from build123d import *

# Parameters (mm, degrees)
SKETCH1_R            = 2.5
SKETCH1_W            = 0.25
SKETCH1_H            = 1
SKETCH1_R_2          = 0.5
BOSS_EXTRUDE1_DEPTH  = 15
SKETCH1_3_R          = 2.5
SKETCH1_3_R_2        = 0.5
BOSS_EXTRUDE2_DEPTH  = 0.8
SKETCH1_5_W          = 0.25
SKETCH1_5_H          = 1
BOSS_EXTRUDE3_DEPTH  = 1.5
SKETCH2_R            = 0.200548898
CUT_EXTRUDE3_DEPTH   = 1.5
BOSS_EXTRUDE4_DEPTH  = 0.5
BOSS_EXTRUDE6_START  = 3
BOSS_EXTRUDE6_DEPTH  = 0.5
SKETCH6_R            = 1.35
BOSS_EXTRUDE7_DEPTH  = 8
BOSS_EXTRUDE9_START  = 4.5
SKETCH9_R            = 0.5
SKETCH9_R_2          = 1.5
BOSS_EXTRUDE9_DEPTH  = 0.5
SKETCH10_R           = 2
SKETCH10_R_2         = 1.5
BOSS_EXTRUDE10_DEPTH = 0.5
FILLET1_R            = 0.5
BOSS_EXTRUDE11_START = -0.5
SKETCH11_R           = 1.5
BOSS_EXTRUDE11_DEPTH = 0.5


with BuildPart() as part:
    # Sketch1 → Boss-Extrude1 (new body)
    # profile 1 of 5: a face of its own
    with BuildSketch(Plane(origin=(0, 0, 0), x_dir=(1, 0, 0), z_dir=(0, 1, 0))):
        with BuildLine():
            Line((-3.31662479, -5), (3.31662479, -5))
            ThreePointArc((3.31662479, -5), (6, 0), (3.31662479, 5))
            Line((3.31662479, 5), (-3.31662479, 5))
            ThreePointArc((-3.31662479, 5), (-6, 0), (-3.31662479, -5))
        make_face()
        Circle(SKETCH1_R, mode=Mode.SUBTRACT)
        with Locations((4, 0)):
            Rectangle(SKETCH1_W, SKETCH1_H, mode=Mode.SUBTRACT)
        with Locations((-4, 0)):
            Rectangle(SKETCH1_W, SKETCH1_H, mode=Mode.SUBTRACT)
    # profile 2 of 5: a face of its own
    with BuildSketch(Plane(origin=(0, 0, 0), x_dir=(1, 0, 0), z_dir=(0, 1, 0))):
        Circle(SKETCH1_R)
        Circle(SKETCH1_R_2, mode=Mode.SUBTRACT)
    # profile 3 of 5: a face of its own
    with BuildSketch(Plane(origin=(0, 0, 0), x_dir=(1, 0, 0), z_dir=(0, 1, 0))):
        with Locations((-4, 0)):
            Rectangle(SKETCH1_W, SKETCH1_H)
    # profile 4 of 5: a face of its own
    with BuildSketch(Plane(origin=(0, 0, 0), x_dir=(1, 0, 0), z_dir=(0, 1, 0))):
        Circle(SKETCH1_R_2)
    # profile 5 of 5: a face of its own
    with BuildSketch(Plane(origin=(0, 0, 0), x_dir=(1, 0, 0), z_dir=(0, 1, 0))):
        with Locations((4, 0)):
            Rectangle(SKETCH1_W, SKETCH1_H)
    extrude(amount=-BOSS_EXTRUDE1_DEPTH)

    # Sketch1<3> → Boss-Extrude2 (add)
    with BuildSketch(Plane(origin=(0, 0, 0), x_dir=(1, 0, 0), z_dir=(0, 1, 0))):
        with Locations(Location((0, 0, 0), (0, 0, 270))):
            Circle(SKETCH1_3_R)
        with Locations(Location((0, 0, 0), (0, 0, 270))):
            Circle(SKETCH1_3_R_2, mode=Mode.SUBTRACT)
    extrude(amount=BOSS_EXTRUDE2_DEPTH)

    # Sketch1<5> → Boss-Extrude3 (add)
    with BuildSketch(Plane(origin=(0, 0, 0), x_dir=(1, 0, 0), z_dir=(0, 1, 0))):
        with Locations((-4, 0)):
            Rectangle(SKETCH1_5_W, SKETCH1_5_H)
    boss_extrude3 = extrude(amount=BOSS_EXTRUDE3_DEPTH)

    # Sketch2 → Cut-Extrude3 (cut)
    with BuildSketch(Plane.ZY.offset(4.125)):
        with Locations((0, 1)):
            Circle(SKETCH2_R)
        with BuildLine():
            Line((-0.5, 1.5), (-0.5, 1))
            ThreePointArc((-0.5, 1), (-0.353553391, 1.353553391), (0, 1.5))
            Line((0, 1.5), (-0.5, 1.5))
        make_face()
        with BuildLine():
            Line((0.5, 1.5), (0, 1.5))
            ThreePointArc((0, 1.5), (0.353553391, 1.353553391), (0.5, 1))
            Line((0.5, 1), (0.5, 1.5))
        make_face()
    cut_extrude3 = extrude(amount=-CUT_EXTRUDE3_DEPTH, mode=Mode.SUBTRACT)

    # Mirror1: Boss-Extrude3, Cut-Extrude3 across plane
    add(boss_extrude3.mirror(Plane(origin=(0, 0, 0), x_dir=(0, 0, 1), z_dir=(1, 0, 0))))
    add(cut_extrude3.mirror(Plane(origin=(0, 0, 0), x_dir=(0, 0, 1), z_dir=(1, 0, 0))), mode=Mode.SUBTRACT)

    # Sketch3 → Boss-Extrude4 (add)
    with BuildSketch(Plane.XZ.offset(15)):
        with BuildLine():
            Line((-5.84848114, -5), (5.84848114, -5))
            ThreePointArc((5.84848114, -5), (5.955621153, -4.955621153), (6, -4.84848114))
            Line((6, -4.84848114), (6, 4.84848114))
            ThreePointArc((6, 4.84848114), (5.955621153, 4.955621153), (5.84848114, 5))
            Line((5.84848114, 5), (-5.84848114, 5))
            ThreePointArc((-5.84848114, 5), (-5.955621153, 4.955621153), (-6, 4.84848114))
            Line((-6, 4.84848114), (-6, -4.84848114))
            ThreePointArc((-6, -4.84848114), (-5.955621153, -4.955621153), (-5.84848114, -5))
        make_face()
    extrude(amount=BOSS_EXTRUDE4_DEPTH)



with BuildPart() as body_2:
    # Sketch7 → Boss-Extrude6 (new body)
    with BuildSketch(Plane.XZ.offset(15.5).offset(BOSS_EXTRUDE6_START)):
        with BuildLine():
            Line((-6, -4.84848114), (-6, 4.84848114))
            ThreePointArc((-6, 4.84848114), (-5.955621153, 4.955621153), (-5.84848114, 5))
            Line((-5.84848114, 5), (5.84848114, 5))
            ThreePointArc((5.84848114, 5), (5.955621153, 4.955621153), (6, 4.84848114))
            Line((6, 4.84848114), (6, -4.84848114))
            ThreePointArc((6, -4.84848114), (5.955621153, -4.955621153), (5.84848114, -5))
            Line((5.84848114, -5), (-5.84848114, -5))
            ThreePointArc((-5.84848114, -5), (-5.955621153, -4.955621153), (-6, -4.84848114))
        make_face()
    extrude(amount=BOSS_EXTRUDE6_DEPTH)


with BuildPart() as part_1:
    add(part.part)

    add(body_2.part)  # Boss-Extrude7 merges body 2
    # Sketch6 → Boss-Extrude7 (add)
    with BuildSketch(Plane.XZ.offset(15.5)):
        with Locations(Location((-4.5, -3.5, 0), (0, 0, 90))):
            Circle(SKETCH6_R)
        with Locations(Location((4.5, 3.5, 0), (0, 0, 90))):
            Circle(SKETCH6_R)
    extrude(amount=BOSS_EXTRUDE7_DEPTH)

    # Sketch9 → Boss-Extrude9 (add)
    with BuildSketch(Plane.XZ.offset(19).offset(BOSS_EXTRUDE9_START)):
        with BuildLine():
            Line((-5.84848114, 5), (5.84848114, 5))
            ThreePointArc((5.84848114, 5), (5.955621153, 4.955621153), (6, 4.84848114))
            Line((6, 4.84848114), (6, -4.84848114))
            ThreePointArc((6, -4.84848114), (5.955621153, -4.955621153), (5.84848114, -5))
            Line((5.84848114, -5), (-5.84848114, -5))
            ThreePointArc((-5.84848114, -5), (-5.955621153, -4.955621153), (-6, -4.84848114))
            Line((-6, -4.84848114), (-6, 4.84848114))
            ThreePointArc((-6, 4.84848114), (-5.955621153, 4.955621153), (-5.84848114, 5))
        make_face()
        with Locations(Location((-4.5, 0, 0), (0, 0, 270))):
            Circle(SKETCH9_R, mode=Mode.SUBTRACT)
        with Locations(Location((4.5, 0, 0), (0, 0, 90))):
            Circle(SKETCH9_R, mode=Mode.SUBTRACT)
        with Locations(Location((0, 0, 0), (0, 0, 270))):
            Circle(SKETCH9_R_2, mode=Mode.SUBTRACT)
    extrude(amount=BOSS_EXTRUDE9_DEPTH)

    # Sketch10 → Boss-Extrude10 (add)
    with BuildSketch(Plane.XZ.offset(24)):
        with Locations(Location((0, 0, 0), (0, 0, 270))):
            Circle(SKETCH10_R)
        with Locations(Location((0, 0, 0), (0, 0, 270))):
            Circle(SKETCH10_R_2, mode=Mode.SUBTRACT)
    extrude(amount=BOSS_EXTRUDE10_DEPTH)

    # Fillet1
    fillet1_edges = [part_1.edges().sort_by_distance(p)[0] for p in [
        (0, -24.5, 2),
    ]]
    fillet(fillet1_edges, radius=FILLET1_R - 0.0001)  # a hair under: the kernel refuses the full size

    # Sketch11 → Boss-Extrude11 (add)
    with BuildSketch(Plane.XZ.offset(24).offset(BOSS_EXTRUDE11_START)):
        with Locations(Location((0, 0, 0), (0, 0, 270))):
            Circle(SKETCH11_R)
    extrude(amount=BOSS_EXTRUDE11_DEPTH)


solid = part_1.part
Geometry: final body of the model. Coordinates: model frame, mm. A direction names the side the tool comes from. Give positions to 0.01 mm unless a question says otherwise; leave off trailing zeros. Write each loop counter-clockwise with the first axis right and the second up, starting at its lowest first coordinate (ties: lowest second). Pieces come first, ordered by that corner, then holes.
(1) Cut plane C-C, the plane y = -17.5. Return loops of the section in (x, z), then the cut area to 3 significant figures.
(2) Cut plane D-D, the plane z = -3.5. Return loops of the section in (x, y), then the cut area to 3 significant figures.
(3) Mould query, pull axis X, two halves, no side actions, for faces 6 (the cylindrical face through (5.7, -16.98, 4.12)), 7 (the flat face through (0, -19, 0)), 8 (the cylindrical face through (-6, -7, 0)), 9 (the cylindrical face through (0.45, -24.25, -1.43)). Classes: released by +X, released by -X, zero draft, split by the parting line, or undercut.
(4) Cut plane A-A, the plane x = 0. Give the number of separate pieces and of enclosed holes in the cut face, then the cut area to 3 significant figures.
(5) Ray query, line 1 (Y direction, x = -1, z = 3.5); line 2 (X direction, y = -23.8, z = 0); line 3 (Y direction, x = 0.5, z = -0.25). Return the intervals inside material, ascending.
(6) Access query for faces 1 (the flat face through (3.875, 0.6, 0)), 2 (the cylindrical face through (4.004, -23.746, -0.065)), 3 (the flat face through (0, -23.5, 0)), 4 (the flat face through (5, -15, 4)), 5 (the flat face through (0, 0, 0)). Directions: +Z, -Z, +X, -X, +Y, -Y. A direction counts if a zero-diameter tool reaches every point of the face in a straight line with its end or side. Return the directions, or none.
(7) First-contact query: P1, Ø1, axis at x = -2.5, z = 3.5, coming from the -Y side; P2, Ø5.5, axis at x = -1, z = 0, coming from the +Y side; P3, Ø2, axis at x = 4.5, z = 2, coming from the +Y side; P4, Ø5, axis at x = -1.5, z = -1.5, coming from the -Y side. Flat tips, straight axial feed; report the tip coordinate or a pass-through.
(8) Cut plane B-B, the plane x = -4.5. Return loops of the section in (y, z), then the cut area to 3 significant figures.
Values follow:
1. outline: circle Ø2.7 at (-4.5, -3.5); circle Ø2.7 at (4.5, 3.5)
1. area: 11.5 mm2
2. outline: (-6, -24) - (6, -24) - (6, -23.5) - (-3.15, -23.5) - (-3.15, -19) - (6, -19) - (6, -18.5) - (-3.15, -18.5) - (-3.15, -15.5) - (6, -15.5) - (6, -15) - (4.87, -15) - (4.87, 0) - (-4.87, 0) - (-4.87, -15) - (-6, -15) - (-6, -15.5) - (-5.85, -15.5) - (-5.85, -18.5) - (-6, -18.5) - (-6, -19) - (-5.85, -19) - (-5.85, -23.5) - (-6, -23.5) - close
2. area: 184 mm2
3. face 6: split by the parting line
3. face 7: zero draft
3. face 8: released by -X
3. face 9: undercut
4. separate pieces: 3
4. enclosed holes: 0
4. area: 169 mm2
5. line 1: y = -24 to -23.5, -19 to -18.5, -15.5 to 0
5. line 2: x = -6 to -5, -4 to 4, 5 to 6
5. line 3: y = -24 to -23.5, -19 to -18.5, -15.5 to 0.8
6. face 1: +Z, -Z, +Y
6. face 2: -Y
6. face 3: none
6. face 4: +Z, +X, +Y
6. face 5: +Y
7. P1: stops at y = -24
7. P2: stops at y = 0.8
7. P3: stops at y = 0
7. P4: stops at y = -24.5
8. outline: (-24, -5) - (-23.5, -5) - (-23.5, -4.85) - (-19, -4.85) - (-19, -5) - (-18.5, -5) - (-18.5, -4.85) - (-15.5, -4.85) - (-15.5, -5) - (-15, -5) - (-15, -3.97) - (0, -3.97) - (0, 3.97) - (-15, 3.97) - (-15, 5) - (-15.5, 5) - (-15.5, -2.15) - (-18.5, -2.15) - (-18.5, 5) - (-19, 5) - (-19, -2.15) - (-23.5, -2.15) - (-23.5, -0.5) - (-24, -0.5) - close; (-24, 0.5) - (-23.5, 0.5) - (-23.5, 5) - (-24, 5) - close
8. area: 154 mm2
